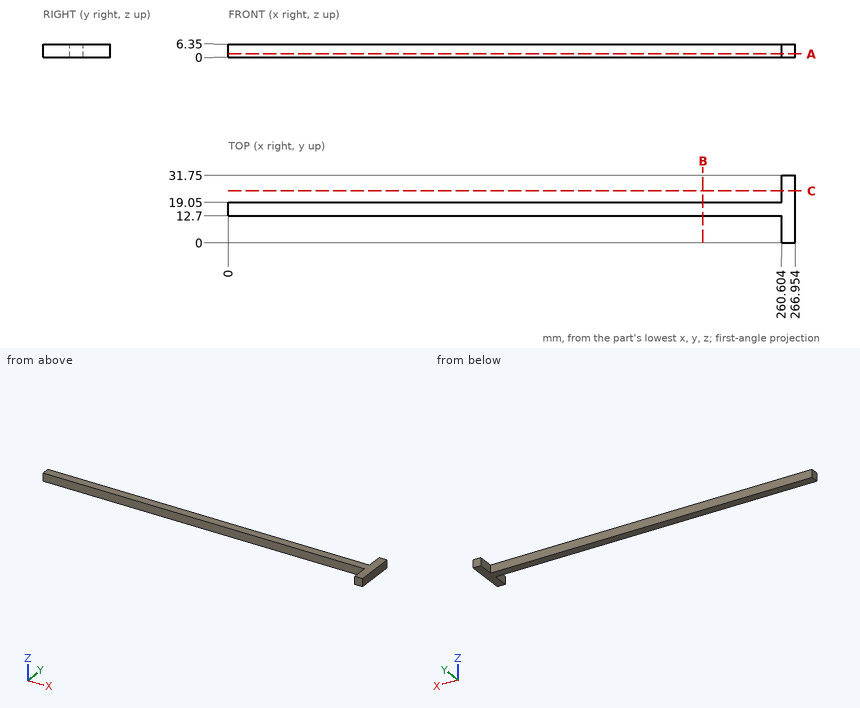
Can you work these out from the drawing? Everything is in mm from the part's minimum corner. Round coordinates to 2 decimals unless told otherwise and drop trailing zeros. Loops run counter-clockwise (first coordinate to the right, second up) from the corner with the lowest first, then second, coordinate; pieces in that order, holes last.
1. If we section it at C-C on y = 24.5: Write out the boundary of the cut face in (x, z), plus the area to 3 significant figures.
Answer list:
outline: (260.6, 0) - (266.95, 0) - (266.95, 6.35) - (260.6, 6.35) - close
area: 40.3 mm2
2. If we section it at B-B on x = 223.5: Write out the boundary of the cut face in (y, z), plus the area to 3 significant figures.
Answer list:
outline: (12.7, 0) - (19.05, 0) - (19.05, 6.35) - (12.7, 6.35) - close
area: 40.3 mm2
3. If I drill on line 1 along X through (y, z) = (22.5, 2); line 2 along Y through (x, z) = (84.5, 2.25), over which ranges is the centre line in solid material (lowest first)?
Answer list:
line 1: x = 260.6 to 266.95
line 2: y = 12.7 to 19.05
4. If we section it at A-A on z = 1.75: Write out the boundary of the cut face in (x, y).
Answer list:
outline: (0, 12.7) - (260.6, 12.7) - (260.6, 0) - (266.95, 0) - (266.95, 31.75) - (260.6, 31.75) - (260.6, 19.05) - (0, 19.05) - close
5. For P1, Ø3, axis at y = 4, z = 3.5, coming from the -X side; P2, Ø3, axis at x = 156, z = 4.5, coming from the +Y side; P3, Ø3, axis at x = 159, z = 2, coming from the -Y side, each with a flat end and sliding along its axis, tell me the tip position at first contact or that it passes through.
Answer list:
P1: stops at x = 260.6
P2: stops at y = 19.05
P3: stops at y = 12.7
